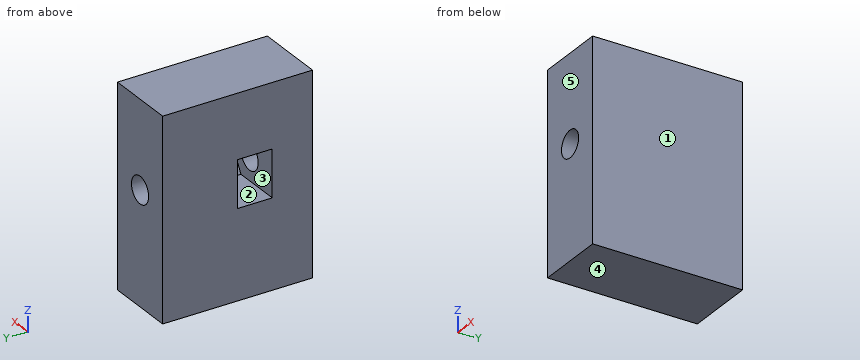
Autodesk Inventor part; units mm, degrees
ref_plane "YZ Plane" through (0, 0, 0) normal (1, 0, 0) x (0, 1, 0)
ref_plane "XZ Plane" through (0, 0, 0) normal (0, 1, 0) x (-1, 0, 0)
ref_plane "XY Plane" through (0, 0, 0) normal (0, 0, 1) x (1, 0, 0)
sketch "Sketch1" plane through (0, 0, 0) normal (0, 1, 0) x (-1, 0, 0)
  line L0 (0, 0) -> (9, 0)
  line L1 (9, 0) -> (9, -25.4)
  line L2 (9, -25.4) -> (0, -25.4)
  line L3 (0, -25.4) -> (0, 0)
  dimension "d0" = 9
  dimension "d1" = 25.4
extrude "Extrusion1" add sketch "Sketch1" along normal blind 19.05
ref_plane "Work Plane1" through (0, 9.525, 0) normal (0, 1, 0) x (1, 0, 0)
sketch "Sketch2" plane through (0, 9.525, 0) normal (0, 1, 0) x (1, 0, 0)
  circle A0 centre (-4.5, 11.1125) radius 3.45 construction
  line L0 (-9, 25.4) -> (-9, 0)
  line L1 (-1.05, 11.1125) -> (-2.775, 8.1247)
  line L2 (-2.775, 8.1247) -> (-9, 8.1247)
  line L3 (-9, 14.1003) -> (-2.775, 14.1003)
  line L4 (-2.775, 14.1003) -> (-1.05, 11.1125)
  line L5 (-9, 8.1247) -> (-9, 14.1003)
  point P0 (0, 0)
  dimension "d4" = 6.9
  dimension "d5" = 4.5
extrude "Extrusion2" cut sketch "Sketch2" against normal blind 4.4
sketch "Sketch3" plane through (0, 0, 0) normal (0, -1, 0) x (1, 0, 0)
  line L0 (-2.775, -8.1247) -> (-9, -8.1247) construction
  line L1 (-9, -14.1003) -> (-2.775, -14.1003) construction
  line L2 (-2.775, -14.1003) -> (-1.05, -11.1125) construction
  line L3 (-1.05, -11.1125) -> (-2.775, -8.1247) construction
  circle A0 centre (-4.5, -11.1125) radius 1.7
  line L4 (-9, -25.4) -> (-9, 0)
  point P0 (0, 0)
  dimension "d8" = 3.4
  dimension "d9" = 4.5
extrude "Extrusion3" cut sketch "Sketch3" against normal through all
properties part number "drop in nut test"
Model file for the job. Use its own axes, mm. Face numbers are marked on the shaded views. A direction names the side the tool comes from. Give positions to 0.01 mm unless a question says otherwise; leave off trailing zeros. Order: outer loops, then holes, each group sorted by start corner. A loop starts at its lowest first (then second) coordinate and runs counter-clockwise, first axis right, second up. Notation, with made-up numbers: (73, 22.5) - (127, 22.5) arc R17 cw to (127, 47.5) - close; hole circle Ø8 at (11.25, 65). An arc over 180 degrees is marked (long way). Write item = value, one per line. Start each with the question number.
1. Cut at D-D, the plane x = -7.25. List the corners of the cut face in (y, z) (3 decimals), and give its area (3 significant figures).
2. Cut at C-C, the plane z = -10.75. List the corners of the cut face in (x, y) (3 decimals), and give its area (3 significant figures).
3. Which spindle directions (+Z, -Z, +X, -X, +Y, -Y) get a long thin tool onto all of the face, cutting with end or side? Do the marked faces 1 and 2. Say none if no direction does.
4. Cut at B-B, the plane y = 4.75. List the corners of the cut face in (x, z).
5. Probe line 1 along Z through (x, y) = (-4.5, 2.7); line 2 along Y through (x, z) = (-2.75, -13) (3 decimals); line 3 along Z through (x, y) = (-3.5, 6). List the from-to ranges inside material, lowest first.
6. Two-plate mould, pull along Z, no slides. Class the marked faces 3, 4 and 5: pulls with the +Z half, pulls with the -Z half, needs draft (parallel to the pull), parting line crosses it, or undercut.
Taken from the geometry:
q1.outline = (0, -25.4) - (19.05, -25.4) - (19.05, 0) - (0, 0) - close; hole (5.125, -14.1) - (9.525, -14.1) - (9.525, -8.125) - (5.125, -8.125) - close
q1.area = 458 mm²
q2.outline = (-9, 0) - (-6.161, 0) - (-6.161, 5.125) - (-9, 5.125) - close; (-9, 9.525) - (-6.161, 9.525) - (-6.161, 19.05) - (-9, 19.05) - close; (-2.839, 0) - (0, 0) - (0, 19.05) - (-2.839, 19.05) - (-2.839, 9.525) - (-1.259, 9.525) - (-1.259, 5.125) - (-2.839, 5.125) - close
q2.area = 88.7 mm²
q3.face_1 = +Z, -Z, +X, +Y, -Y
q3.face_2 = -X
q4.outline = (-9, -25.4) - (0, -25.4) - (0, 0) - (-9, 0) - close; hole circle Ø3.4 at (-4.5, -11.11)
q5.line_1 = -25.4 to -12.81, -9.41 to 0
q5.line_2 = 0 to 5.125, 9.525 to 19.05
q5.line_3 = -25.4 to -14.1, -8.12 to 0
q6.face_3 = undercut
q6.face_4 = pulls with the -Z half
q6.face_5 = needs draft
